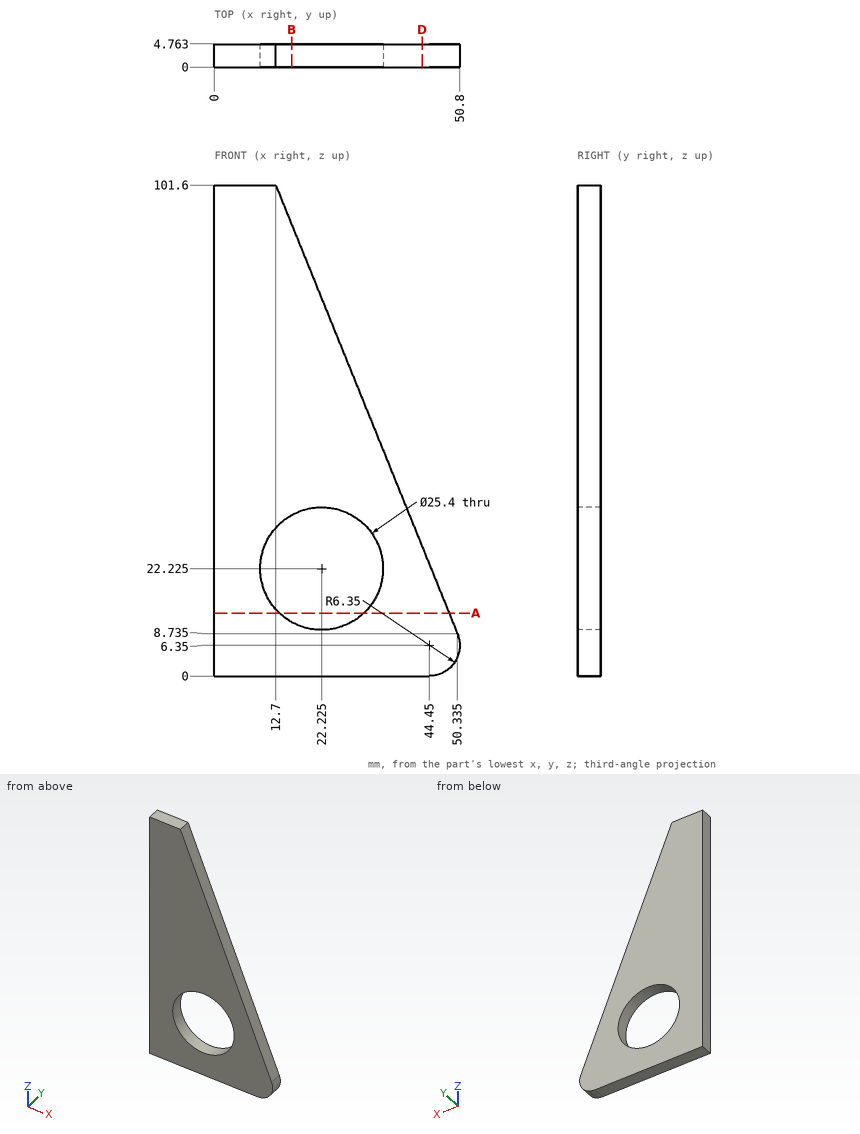
For this review, use the dimensioned drawing (mm, ordinates from the lowest corner) and the shaded views. Round coordinates to 2 decimals unless told otherwise and drop trailing zeros. Order: outer loops, then holes, each group sorted by start corner. A loop starts at its lowest first (then second) coordinate and runs counter-clockwise, first axis right, second up.
1) Consider section B-B (x = 16). State the section outline as (y, z) points (1 decimal).
The answers:
outline: (0, 0) - (4.8, 0) - (4.8, 11.2) - (0, 11.2) - close; (0, 33.3) - (4.8, 33.3) - (4.8, 93.5) - (0, 93.5) - close
2) Clearance check with flat-ended pins moving along their axes: pin 1 Ø1.5 at (y, z) = (1, 15.5) entering from +X; pin 2 Ø2 at (x, y) = (22, 2) entering from +Z. State where each tip first meets the part, or that it passes through.
The answers:
pin 1: stops at x = 47.9
pin 2: stops at z = 81.12
3) Consider section A-A (z = 13). State the section outline as (x, y) points, plus the area to 3 significant figures.
The answers:
outline: (0, 0) - (13.5, 0) - (13.5, 4.76) - (0, 4.76) - close; (30.95, 0) - (48.61, 0) - (48.61, 4.76) - (30.95, 4.76) - close
area: 148 mm2
4) Consider section D-D (x = 43). State the section outline as (y, z) points (1 decimal).
The answers:
outline: (0, 0) - (4.8, 0) - (4.8, 26.8) - (0, 26.8) - close
5) For L1, parallel to X at y = 2, z = 28 (1 decimal); L2, parallel to Z at x = 27, y = 3.8 (1 decimal); L3, parallel to Z at x = 15, y = 1.9 (1 decimal), list the stretches that pass through material, from the lowest coordinate up.
The answers:
L1: x = 0 to 10.9, 33.5 to 42.5
L2: z = 0 to 10.5, 34 to 66.3
L3: z = 0 to 11.8, 32.7 to 95.9
